from build123d import *

# Parameters (mm, degrees)
F1_DEPTH = 25.4
F3_DEPTH = 25.4
F4_R     = 15.875
F5_DEPTH = 76.2


with BuildPart() as f1:
    # F0 (on Top) → F1 (new body)
    with BuildSketch(Plane.XY):
        with BuildLine():
            Line((76.2, 19.05), (0, 19.05))
            ThreePointArc((0, 19.05), (-19.05, 0), (0, -19.05))
            Line((0, -19.05), (76.2, -19.05))
            ThreePointArc((76.2, -19.05), (95.25, 0), (76.2, 19.05))
        make_face()
    extrude(amount=F1_DEPTH)

    # F2 (on face) → F3 (join)
    with BuildSketch(Plane.XY.offset(25.4)):
        with BuildLine():
            Line((76.2, 12.7), (0, 12.7))
            ThreePointArc((0, 12.7), (-12.7, 0), (0, -12.7))
            Line((0, -12.7), (76.2, -12.7))
            ThreePointArc((76.2, -12.7), (63.5, 0), (76.2, 12.7))
        make_face()
        with BuildLine():
            ThreePointArc((88.9, 0), (85.180256, 8.980256), (76.2, 12.7))
            ThreePointArc((76.2, 12.7), (63.5, 0), (76.2, -12.7))
            ThreePointArc((76.2, -12.7), (85.180256, -8.980256), (88.9, 0))
        make_face()
    extrude(amount=F3_DEPTH)

    # F4 (on face) → F5 (join)
    with BuildSketch(Plane(origin=(0, 0, 0), x_dir=(1, 0, 0), z_dir=(0, 0, -1))):
        with Locations((38.1, 0)):
            Circle(F4_R)
    extrude(amount=F5_DEPTH)


solid = f1.part
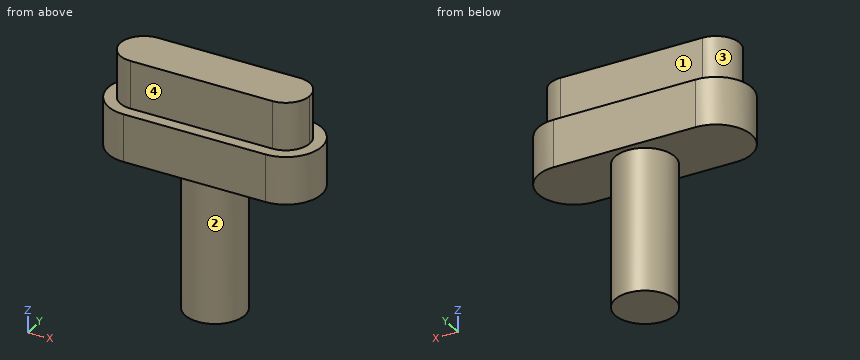
Geometry: final body of the model. Coordinates: model frame, mm. Face numbers are marked on the shaded views. A direction names the side the tool comes from. Round coordinates to 2 decimals unless told otherwise and drop trailing zeros. Order: outer loops, then holes, each group sorted by start corner. A loop starts at its lowest first (then second) coordinate and runs counter-clockwise, first axis right, second up.
Q1. Access query for the marked faces 1, 2, 3 and 4. Directions: +Z, -Z, +X, -X, +Y, -Y. A direction counts if a zero-diameter tool reaches every point of the face in a straight line with its end or side. Return the directions, or none.
Result sheet:
face 1: +Z, +X, -X, +Y
face 2: -Z
face 3: +Z, -X
face 4: +Z, +X, -X, -Y
Q2. Pin query (flat end, axial travel): pin 1 (20.5 mm diameter, centred on x = 53.5, z = 40.5, fed in from +Y); pin 2 (12 mm diameter, centred on y = -1.5, z = -22.5, fed in from -X) (3 decimals); pin 3 (5 mm diameter, centred on x = 1, y = 15, fed in from -Z). Return the tip coordinate at first contact, or that it passes through.
Result sheet:
pin 1: stops at y = 12.7
pin 2: stops at x = 22.225
pin 3: stops at z = 0
Q3. Section A-A, the plane x = 66. Output: boundary loops of the cut face in (y, z).
Result sheet:
outline: (-19.05, 0) - (19.05, 0) - (19.05, 25.4) - (12.7, 25.4) - (12.7, 50.8) - (-12.7, 50.8) - (-12.7, 25.4) - (-19.05, 25.4) - close
Q4. Section B-B, the plane y = 5. Output: boundary loops of the cut face in (x, z), and give its area (3 significant figures).
Result sheet:
outline: (-18.38, 0) - (23.03, 0) - (23.03, -76.2) - (53.17, -76.2) - (53.17, 0) - (94.58, 0) - (94.58, 25.4) - (87.87, 25.4) - (87.87, 50.8) - (-11.67, 50.8) - (-11.67, 25.4) - (-18.38, 25.4) - close
area: 7,690 mm2
Q5. Material intervals for probe 1 along Z at (x, y) = (19.5, -9); probe 2 along X at (y, z) = (0.5, -47); probe 3 along Y at (x, z) = (18, 44), sorted ascending.
Result sheet:
probe 1: z = 0 to 50.8
probe 2: x = 22.23 to 53.97
probe 3: y = -12.7 to 12.7
Q6. Section D-D, the plane x = 38.1. Output: boundary loops of the cut face in (y, z) (3 decimals), and give its area (3 significant figures).
Result sheet:
outline: (-19.05, 0) - (-15.875, 0) - (-15.875, -76.2) - (15.875, -76.2) - (15.875, 0) - (19.05, 0) - (19.05, 25.4) - (12.7, 25.4) - (12.7, 50.8) - (-12.7, 50.8) - (-12.7, 25.4) - (-19.05, 25.4) - close
area: 4,030 mm2
Q7. Section C-C, the plane z = -23. Output: boundary loops of the cut face in (x, y) (3 decimals), and give its area (3 significant figures).
Result sheet:
outline: circle Ø31.75 at (38.1, 0)
area: 792 mm2
